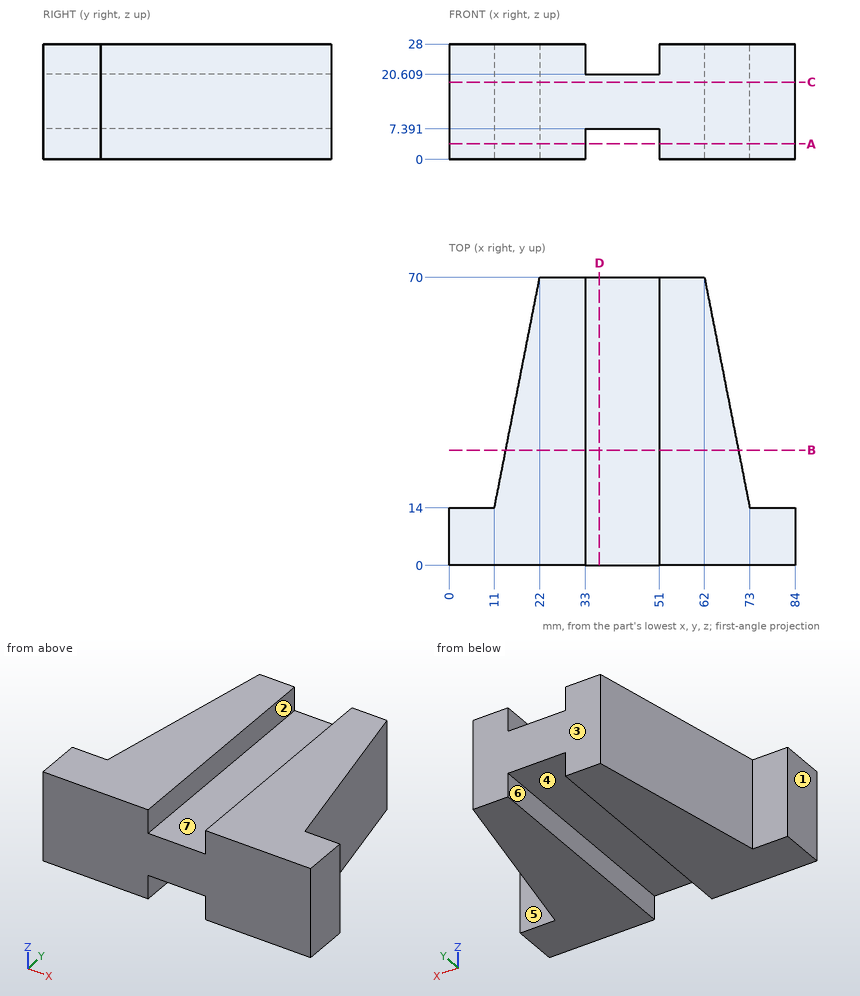
Input: dimensioned drawing with shaded views. Units: mm. Origin: part minimum x, y, z. A direction names the side the tool comes from. Round coordinates to 2 decimals unless told otherwise and drop trailing zeros. Loops run counter-clockwise (first coordinate to the right, second up) from the corner with the lowest first, then second, coordinate; pieces in that order, holes last. Notation, with made-up numbers: M 47,21 L 102,21 A11 cw 102,25 Z; hole C 7.5,85.25 d5. An arc over 180 degrees is marked long. Return JSON: item names as keys, results as strings. Group by question number.
1. Reachability of the marked faces 5, 6 and 7 from +Z, -Z, +X, -X, +Y, -Y: full face, straight path, thin tool, end or side. Return the list, or none.
2. Section query D-D on x = 36.5. Output: boundary loops of the cut face in (y, z), and give its area (3 significant figures).
3. Section query A-A on z = 3.75. Output: boundary loops of the cut face in (x, y), and give its area (3 significant figures).
4. Section query B-B on y = 28. Output: boundary loops of the cut face in (x, z).
5. Material intervals for line 1 along X through (y, z) = (5, 5.25); line 2 along X through (y, z) = (33.5, 24.75); line 3 along Z through (x, y) = (40, 54), sorted ascending. Write a range as from..to.
6. Pin query (flat end, axial travel): pin 1 (9 mm diameter, centred on x = 39.5, y = 31, fed in from +Z); pin 2 (3.5 mm diameter, centred on y = 38.5, z = 24, fed in from +X); pin 3 (12 mm diameter, centred on y = 49.5, z = 9.5, fed in from -X). Return the tip coordinate at first contact, or that it passes through.
7. Mould query, pull axis X, two halves, no side actions, for the marked faces 1, 2, 3 and 4. Classes: released by +X, released by -X, zero draft, split by the parting line, or undercut.
8. Section query C-C on z = 18.75. Output: boundary loops of the cut face in (x, y).
Checks:
{
 "1": {"face 5": "+Z, -Z, +X, +Y", "face 6": "-Z, +Y, -Y", "face 7": "+Z, +Y, -Y"},
 "2": {"outline": "M 0,7.39 L 70,7.39 L 70,20.61 L 0,20.61 Z", "area": "925 mm²"},
 "3": {"outline": "M 0,0 L 33,0 L 33,70 L 22,70 L 11,14 L 0,14 Z; M 51,0 L 84,0 L 84,14 L 73,14 L 62,70 L 51,70 Z", "area": "2,770 mm²"},
 "4": {"outline": "M 13.75,0 L 33,0 L 33,7.39 L 51,7.39 L 51,0 L 70.25,0 L 70.25,28 L 51,28 L 51,20.61 L 33,20.61 L 33,28 L 13.75,28 Z"},
 "5": {"line 1": "x = 0..33, 51..84", "line 2": "x = 14.83..33, 51..69.17", "line 3": "z = 7.39..20.61"},
 "6": {"pin 1": "stops at z = 20.61", "pin 2": "stops at x = 68.53", "pin 3": "stops at x = 16.79"},
 "7": {"face 1": "released by -X", "face 2": "undercut", "face 3": "zero draft", "face 4": "undercut"},
 "8": {"outline": "M 0,0 L 84,0 L 84,14 L 73,14 L 62,70 L 22,70 L 11,14 L 0,14 Z"}
}
